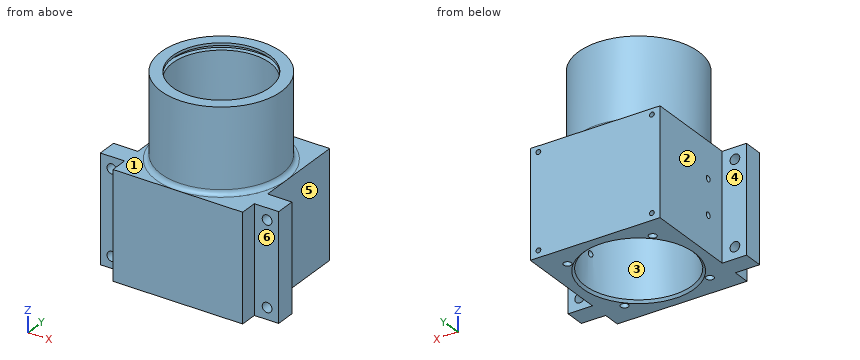
```python
from build123d import *

# Parameters (mm, degrees)
SKETCH_1_W                  = 56
SKETCH_1_H                  = 56
EXTRUDE_1_DEPTH             = 82
SKETCH_4_W                  = 56
SKETCH_4_H                  = 56
SKETCH_4_R                  = 26
CUT_EXTRUDE_1_DEPTH         = 36
HOLE_WIZARD_M4_1_D          = 3.3
HOLE_WIZARD_M4_1_DEPTH      = 10.1
HOLE_WIZARD_M4_1_TIP        = 0.991420021
SKETCH_15_W                 = 23
SKETCH_15_H                 = 1.9
FILLET_1_R                  = 2
CHAMFER_2_SIZE              = 1
HOLE_WIZARD_M2_5_1_D        = 2.05
HOLE_WIZARD_M2_5_1_DEPTH    = 7.25
HOLE_WIZARD_M2_5_1_TIP      = 0.615882135
SKETCH_19_W                 = 10.5
SKETCH_19_H                 = 46
EXTRUDE_2_DEPTH             = 16
HOLE_WIZARD_M5_1_D          = 4.2
HOLE_WIZARD_M3_1_AT_2_COUNT = 2
HOLE_WIZARD_M3_1_AT_2_PITCH = 15
CUT_EXTRUDE_2_REACH         = 96.817
SKETCH_25_W                 = 10.5
SKETCH_25_H                 = 7.5


with BuildPart() as part:
    # 草图1 → 凸台-拉伸1 (new body)
    with BuildSketch(Plane.XY):
        Rectangle(SKETCH_1_W, SKETCH_1_H)
    extrude(amount=EXTRUDE_1_DEPTH)

    # 草图3 → 切除-旋转2 (revolve, cut)
    with BuildSketch(Plane(origin=(0, 0, 0), x_dir=(0, 0, -1), z_dir=(1, 0, 0)), mode=Mode.PRIVATE) as cut_revolve_2_sk:
        Polygon((-82, 0), (0, 0), (0, 23), (-52, 23), (-52, 20), (-56, 20), (-56, 21), (-82, 21), align=None)
    revolve(cut_revolve_2_sk.sketch.rotate(Axis((0, 0, -5.719261836), (0, 0, 1)), 90), axis=Axis((0, 0, -5.719261836), (0, 0, 1)), mode=Mode.SUBTRACT)

    # 草图4 → 切除-拉伸1 (cut)
    with BuildSketch(Plane.XY.offset(82)):
        Rectangle(SKETCH_4_W, SKETCH_4_H)
        Circle(SKETCH_4_R, mode=Mode.SUBTRACT)
    extrude(amount=-CUT_EXTRUDE_1_DEPTH, mode=Mode.SUBTRACT)

    # M4 螺纹孔1
    with Locations(Plane(origin=(0, 0, 0), x_dir=(-1, 0, 0), z_dir=(0, 0, -1))):
        with Locations((18.384776311, 18.384776311), (18.384776311, -18.384776311), (-18.384776311, -18.384776311), (-18.384776311, 18.384776311)):
            Hole(HOLE_WIZARD_M4_1_D / 2, depth=HOLE_WIZARD_M4_1_DEPTH)
            with Locations((0, 0, -(HOLE_WIZARD_M4_1_DEPTH + HOLE_WIZARD_M4_1_TIP / 2))):  # 118° drill point
                Cone(0, HOLE_WIZARD_M4_1_D / 2, HOLE_WIZARD_M4_1_TIP, mode=Mode.SUBTRACT)

    # 草图15 → 切除-旋转3 (revolve, cut)
    with BuildSketch(Plane(origin=(0, 0, 0), x_dir=(1, 0, 0), z_dir=(0, 1, 0))):
        with Locations((-11.5, -79.95)):
            Rectangle(SKETCH_15_W, SKETCH_15_H)
    revolve(axis=Axis((0, 0, 0), (0, 0, 1)), mode=Mode.SUBTRACT)

    # 圆角1
    fillet_1_edges = [part.edges().sort_by_distance(p)[0] for p in [
        (-26, 0, 46),
    ]]
    fillet(fillet_1_edges, radius=FILLET_1_R - 0.0001)  # a hair under: the kernel refuses the full size

    # 倒角2
    chamfer_2_edges = [part.edges().sort_by_distance(p)[0] for p in [
        (23, 0, 0),
    ]]
    chamfer(chamfer_2_edges, length=CHAMFER_2_SIZE)

    # M2.5 螺纹孔1
    with Locations(Plane(origin=(0, 28, 0), x_dir=(1, 0, 0), z_dir=(0, 1, 0))):
        with Locations((24.5, -3), (-24.5, -43.5), (-24.5, -3), (24.5, -43.5)):
            Hole(HOLE_WIZARD_M2_5_1_D / 2, depth=HOLE_WIZARD_M2_5_1_DEPTH)
            with Locations((0, 0, -(HOLE_WIZARD_M2_5_1_DEPTH + HOLE_WIZARD_M2_5_1_TIP / 2))):  # 118° drill point
                Cone(0, HOLE_WIZARD_M2_5_1_D / 2, HOLE_WIZARD_M2_5_1_TIP, mode=Mode.SUBTRACT)

    # 草图19 → 凸台-拉伸2 (add)
    with BuildSketch(Plane.XZ.offset(28)):
        with Locations((33.25, 23)):
            Rectangle(SKETCH_19_W, SKETCH_19_H)
        with Locations((-33.25, 23)):
            Rectangle(SKETCH_19_W, SKETCH_19_H)
    extrude(amount=-EXTRUDE_2_DEPTH)

    # M5 螺纹孔1 (through all)
    with Locations(Plane(origin=(0, -28, 0), x_dir=(-1, 0, 0), z_dir=(0, -1, 0))):
        with Locations((33.5, -5), (-33.5, -41), (-33.5, -5), (33.5, -41)):
            Hole(HOLE_WIZARD_M5_1_D / 2)

    # 草图24 → M3 螺纹孔1 (revolve, cut)
    with BuildSketch(Plane(origin=(28, -3, 30.5), x_dir=(0, 0, -1), z_dir=(0, 1, 0))):
        Polygon((0, 0), (0, 6.251075774), (1.25, 5.5), (1.25, 0), align=None)
    hole_wizard_m3_1 = revolve(axis=Axis((34.35, -3, 30.5), (-1, 0, 0)), mode=Mode.SUBTRACT)

    # M3 螺纹孔1 at 2: M3 螺纹孔1 ×2
    with Locations(*[(0, 0, -i * HOLE_WIZARD_M3_1_AT_2_PITCH) for i in range(1, HOLE_WIZARD_M3_1_AT_2_COUNT)]):
        add(hole_wizard_m3_1, mode=Mode.SUBTRACT)

    # 草图25 → 切除-拉伸2 (cut, up to next)
    with BuildSketch(Plane(origin=(0, 0, 0), x_dir=(-1, 0, 0), z_dir=(0, 0, -1)), mode=Mode.PRIVATE) as cut_extrude_2_sk1:
        with Locations((-33.25, -24.25)):
            Rectangle(SKETCH_25_W, SKETCH_25_H)
    cut_extrude_2_tool1 = extrude(cut_extrude_2_sk1.sketch, amount=-CUT_EXTRUDE_2_REACH, mode=Mode.PRIVATE) & part.part
    cut_extrude_2 = cut_extrude_2_tool1.solids().sort_by_distance((33.25, -24.25, 0))[0]
    add(cut_extrude_2, mode=Mode.SUBTRACT)

    # 镜向1: M3 螺纹孔1, 切除-拉伸2 across plane
    add(hole_wizard_m3_1.mirror(Plane(origin=(0, 0, 0), x_dir=(0, 0, 1), z_dir=(1, 0, 0))), mode=Mode.SUBTRACT)
    add(cut_extrude_2.mirror(Plane(origin=(0, 0, 0), x_dir=(0, 0, 1), z_dir=(1, 0, 0))), mode=Mode.SUBTRACT)

    # 镜向1 copy 1 sketch → 镜向1 copy 1 (revolve, cut)
    with BuildSketch(Plane(origin=(-28, -3, 15.5), x_dir=(0, 0, -1), z_dir=(0, 1, 0))):
        Polygon((0, 0), (0, -6.251075774), (1.25, -5.5), (1.25, 0), align=None)
    revolve(axis=Axis((-34.35, -3, 15.5), (-1, 0, 0)), mode=Mode.SUBTRACT)


solid = part.part
```
Model file for the job. Use its own axes, mm. Face numbers are marked on the shaded views. A direction names the side the tool comes from. Coordinates: 2 decimals unless noted, no trailing zeros. Write each loop counter-clockwise with the first axis right and the second up, starting at its lowest first coordinate (ties: lowest second). Pieces come first, ordered by that corner, then holes. Notation, with made-up numbers: (69.5, 85) - (87.5, 85) arc R23 cw to (87.5, 102) - close; hole circle Ø11 at (56, -8). An arc over 180 degrees is marked (long way). One line per item, written item: value. Start each with the question number.
1. Probe line 1 (Z direction, x = -33.5, y = -14.25); line 2 (Z direction, x = -24, y = 22); line 3 (Y direction, x = 0, z = 68.5). List the from-to ranges inside material, lowest first. Write a range as from..to.
2. Flat gauge pins, fed straight in: pin 1 (4 mm diameter, centred on y = -3, z = 30.5, fed in from -X); pin 2 (5.5 mm diameter, centred on x = -33.5, z = 41, fed in from +Y); pin 3 (4 mm diameter, centred on y = -12.5, z = 69, fed in from +X). Where does each tip first touch, or does it go through?
3. Slice it at A-A (z = 41). Write the cut outline in (x, y).
4. Tool access for the marked faces 4, 5 and 6: list every direction of +Z, -Z, +X, -X, +Y, -Y with a clear straight run to the whole face (end or side of a thin tool).
5. Slice it at D-D (z = 53.5). Write the cut outline in (x, y), plus the area to 3 significant figures.
6. Mould opens along X. For the marked faces 1, 2 and 3 say: released by +X, released by -X, zero draft, split by the parting line, or undercut.
Answers below:
1. line 1: z = 0..2.9, 7.1..38.9, 43.1..46
1. line 2: z = 0..2.11, 3.89..42.61, 44.39..46
1. line 3: y = -26..-21, 21..26
2. pin 1: stops at x = -28
2. pin 2: stops at y = -12
2. pin 3: stops at x = 23.79
3. outline: (-38.5, -20.5) - (-35.6, -20.5) - (-35.6, -12) - (-38.5, -12) - close; (-31.4, -20.5) - (-28, -20.5) - (-28, -28) - (28, -28) - (28, -20.5) - (31.4, -20.5) - (31.4, -12) - (28, -12) - (28, 28) - (-28, 28) - (-28, -12) - (-31.4, -12) - close; (35.6, -20.5) - (38.5, -20.5) - (38.5, -12) - (35.6, -12) - close; hole circle Ø46 at (0, 0)
4. face 4: +Z, -Z, -X, +Y
4. face 5: +Z, -Z, +X, +Y
4. face 6: +Z, -Z, +X, -Y
5. outline: circle Ø52 at (0, 0); hole circle Ø40 at (0, 0)
5. area: 867 mm^2
6. face 1: zero draft
6. face 2: released by -X
6. face 3: undercut
